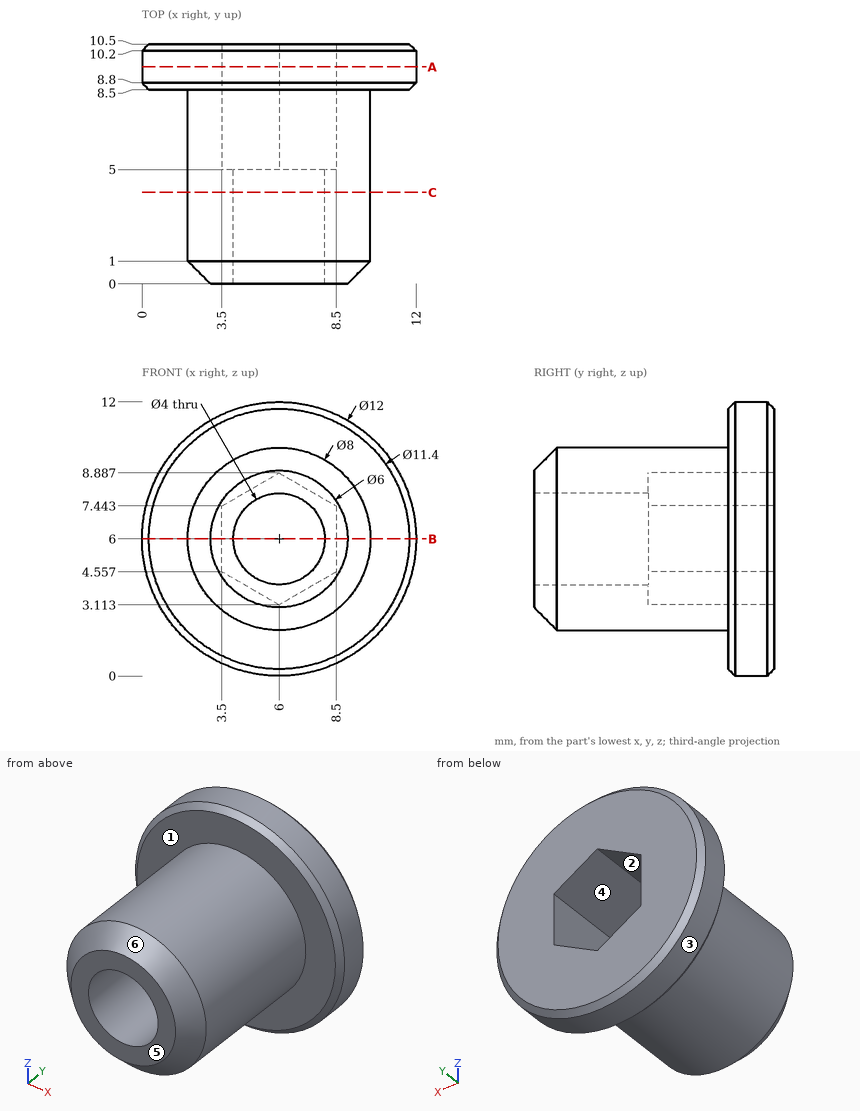
Could you check a few things on this drawing? It's one solid part, dimensions in mm from its lowest x, y, z. A direction names the side the tool comes from. Round coordinates to 2 decimals unless told otherwise and drop trailing zeros. Loops run counter-clockwise (first coordinate to the right, second up) from the corner with the lowest first, then second, coordinate; pieces in that order, holes last.
Q1. I want a section at A-A (y = 9.5). Write out the boundary of the cut face in (x, z).
Q2. For P1, Ø3, axis at x = 8, y = 3.5, coming from the -Z side; P2, Ø2, axis at y = 1.5, z = 10.5, coming from the +X side (1 decimal); P3, Ø3, axis at x = 6, z = 6, coming from the -Y side (3 decimals); P4, Ø1, axis at y = 6, z = 7, coming from the +X side, each with a flat end and sliding along its axis, tell me the tip position at first contact or that it passes through.
Q3. I want a section at C-C (y = 4). Write out the boundary of the cut face in (x, z), and give its area (3 significant figures).
Q4. Thinking about a two-plate mould opening in Z: for the marked faces 4, 5 and 6, which applies, pulls with the +Z half, pulls with the -Z half, needs draft (parallel to the pull), parting line crosses it, or undercut?
Q5. On a 3-axis mill with a long thin cutter (end or side, diameter ignored), from which of +Z, -Z, +X, -X, +Y, -Y can I reach the whole of each face in a straight line? I mean the marked faces 1, 2 and 3. Say none if no direction works.
Q6. Please list where these lines run through material, in increasing order: L1, parallel to X at y = 9, z = 6; L2, parallel to X at y = 3.5, z = 6.
Q7. I want a section at B-B (z = 6). Write out the boundary of the cut face in (x, y).
Answer below:
1. outline: circle Ø12 at (6, 6); hole (3.5, 4.56) - (6, 3.11) - (8.5, 4.56) - (8.5, 7.44) - (6, 8.89) - (3.5, 7.44) - close
2. P1: stops at z = 2.03
2. P2: stops at x = 7.9
2. P3: passes through
2. P4: stops at x = 9.97
3. outline: circle Ø8 at (6, 6); hole circle Ø4 at (6, 6)
3. area: 37.7 mm2
4. face 4: undercut
4. face 5: needs draft
4. face 6: parting line crosses it
5. face 1: -Y
5. face 2: +Y
5. face 3: +Y, -Y
6. L1: x = 0 to 3.5, 8.5 to 12
6. L2: x = 2 to 4, 8 to 10
7. outline: (0, 8.8) - (0.3, 8.5) - (2, 8.5) - (2, 1) - (3, 0) - (4, 0) - (4, 5) - (3.5, 5) - (3.5, 10.5) - (0.3, 10.5) - (0, 10.2) - close; (8, 0) - (9, 0) - (10, 1) - (10, 8.5) - (11.7, 8.5) - (12, 8.8) - (12, 10.2) - (11.7, 10.5) - (8.5, 10.5) - (8.5, 5) - (8, 5) - close
